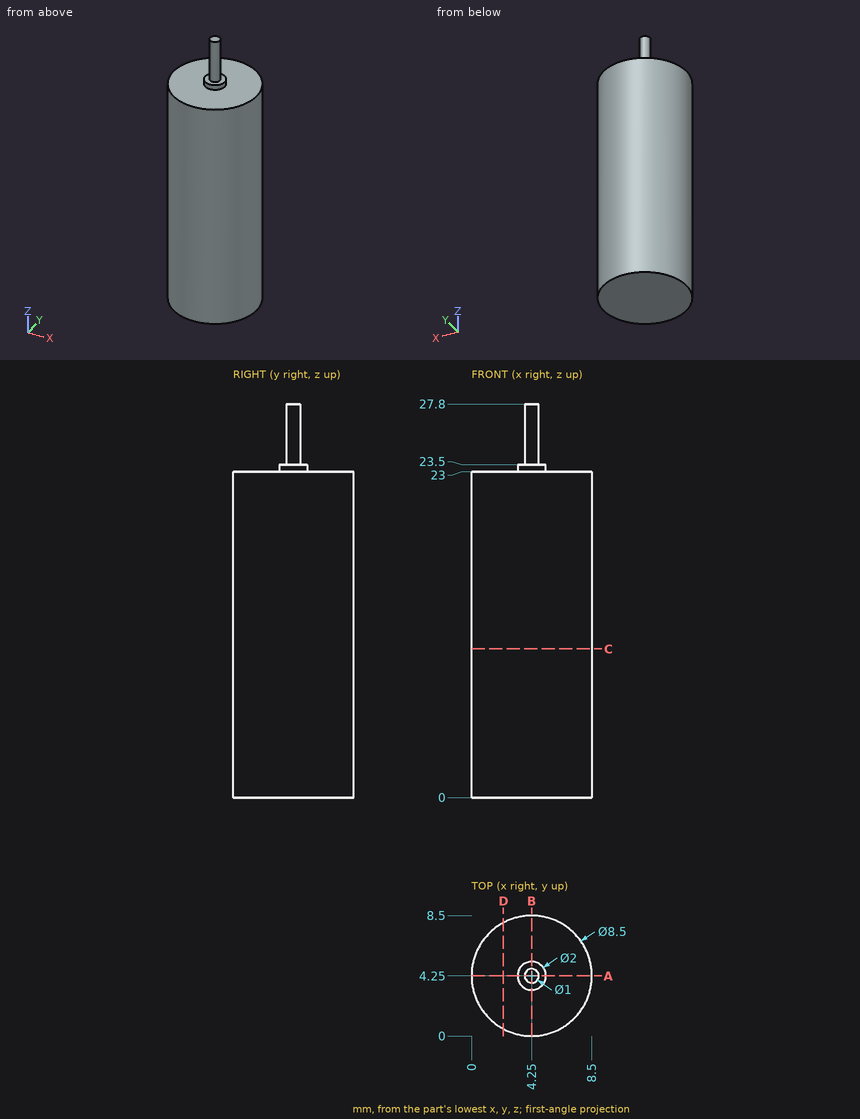
Part print with two shaded views. Sizes in mm from the minimum x, y, z corner. Give positions to 0.01 mm unless a question says otherwise; leave off trailing zeros. Order: outer loops, then holes, each group sorted by start corner. A loop starts at its lowest first (then second) coordinate and runs counter-clockwise, first axis right, second up.
(1) Saw through at D-D, the plane x = 2.25. Give the cut face in (y, z).
(2) Saw through at C-C, the plane z = 10.5. Give the cut face in (x, y).
(3) Drill centre lines: L1, parallel to Z at x = 5.75, y = 1.25; L2, parallel to Z at x = 5, y = 4; L3, parallel to X at y = 2.5, z = 11.25. Where is each one in solid material? Low to high.
(4) Saw through at A-A, the plane y = 4.25. Give the cut face in (x, z), then the cut area to 3 significant figures.
(5) Flat gauge pins, fed straight in: pin 1 (1 mm diameter, centred on y = 4.5, z = 18, fed in from +X); pin 2 (1.5 mm diameter, centred on x = 3, z = 22, fed in from +Y); pin 3 (1 mm diameter, centred on x = 1, z = 3, fed in from -Y). Where does each tip first touch, or does it go through?
Results found:
1. outline: (0.5, 0) - (8, 0) - (8, 23) - (0.5, 23) - close
2. outline: circle Ø8.5 at (4.25, 4.25)
3. L1: z = 0 to 23
3. L2: z = 0 to 23.5
3. L3: x = 0.38 to 8.12
4. outline: (0, 0) - (8.5, 0) - (8.5, 23) - (5.25, 23) - (5.25, 23.5) - (4.75, 23.5) - (4.75, 27.8) - (3.75, 27.8) - (3.75, 23.5) - (3.25, 23.5) - (3.25, 23) - (0, 23) - close
4. area: 201 mm2
5. pin 1: stops at x = 8.5
5. pin 2: stops at y = 8.47
5. pin 3: stops at y = 1.01
